The figure shows three views and two pictorial views of one solid part (mm, origin at its lowest corner). Answer the questions. Coordinates: 2 decimals unless noted, no trailing zeros. Loops run counter-clockwise (first coordinate to the right, second up) from the corner with the lowest first, then second, coordinate; pieces in that order, holes last.
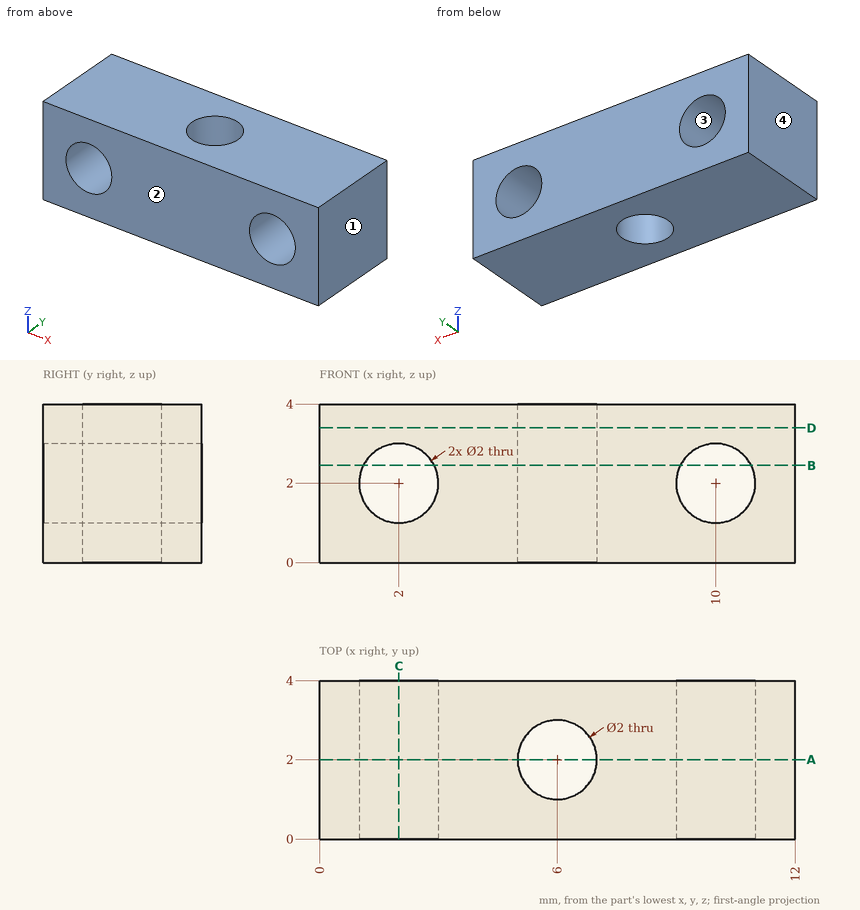
Q1. A cutting plane is placed at B-B (z = 2.45). Give the vertices of the cut face in (x, y).
Findings below:
outline: (0, 0) - (1.11, 0) - (1.11, 4) - (0, 4) - close; (2.89, 0) - (9.11, 0) - (9.11, 4) - (2.89, 4) - close; (10.89, 0) - (12, 0) - (12, 4) - (10.89, 4) - close; hole circle Ø2 at (6, 2)
Q2. A cutting plane is placed at D-D (z = 3.4). Give the vertices of the cut face in (x, y), then the cut area to 3 significant figures.
Findings below:
outline: (0, 0) - (12, 0) - (12, 4) - (0, 4) - close; hole circle Ø2 at (6, 2)
area: 44.9 mm2
Q3. A cutting plane is placed at A-A (y = 2). Give the vertices of the cut face in (x, z), then the cut area to 3 significant figures.
Findings below:
outline: (0, 0) - (5, 0) - (5, 4) - (0, 4) - close; (7, 0) - (12, 0) - (12, 4) - (7, 4) - close; hole circle Ø2 at (2, 2); hole circle Ø2 at (10, 2)
area: 33.7 mm2
Q4. A cutting plane is placed at C-C (x = 2). Give the vertices of the cut face in (y, z), then the cut area to 3 significant figures.
Findings below:
outline: (0, 0) - (4, 0) - (4, 1) - (0, 1) - close; (0, 3) - (4, 3) - (4, 4) - (0, 4) - close
area: 8.00 mm2
Q5. Straight lines are drawn through the part: probe 1 along X at (y, z) = (2.5, 2); probe 2 along X at (y, z) = (3.85, 1.8); probe 3 along Y at (x, z) = (6, 1.05). For each, find the intervals that lie inside material, in ascending order.
Findings below:
probe 1: x = 0 to 1, 3 to 5.13, 6.87 to 9, 11 to 12
probe 2: x = 0 to 1.02, 2.98 to 9.02, 10.98 to 12
probe 3: y = 0 to 1, 3 to 4
Q6. Flat-ended cylindrical pins translate along their axes: pin 1 Ø1.2 at (x, y) = (6, 2) entering from -Z; pin 2 Ø2 at (y, z) = (3.5, 2.5) entering from -X. Find the tip coordinate at first contact, or state that the pin passes through.
Findings below:
pin 1: passes through
pin 2: stops at x = 0
Q7. Determine the mould class of the marked faces 1, 2, 3 and 4 for opening direction X: +X half, -X half, draft (parallel to the pull), parting line (faces both ways), or undercut.
Findings below:
face 1: +X half
face 2: draft
face 3: undercut
face 4: -X half
